Can you work these out from the model? Positions are in its coordinate system, mm. A direction names the side the tool comes from. Round coordinates to 2 decimals unless told otherwise and drop trailing zeros. Order: outer loops, then holes, each group sorted by start corner. A loop starts at its lowest first (then second) coordinate and runs counter-clockwise, first axis right, second up. Notation, with made-up numbers: (85.5, -9) -> (96.5, -9) arc R7 ccw to (96.5, 3) -> close; hole circle Ø11 at (-19, 31.25). An arc over 180 degrees is marked (long way). Use a Markdown table: item, result. Add a question column.
Q1. If we section it at D-D on y = 1.5: Give the number of separate pieces and of enclosed holes in the cut face, plus the area to 3 significant figures.
Q2. I'm going to push flat-ended pins straight in: pin 1 Ø3 at (y, z) = (7.5, 9) entering from +X; pin 2 Ø6 at (x, z) = (17.15, 0) entering from +Y; pin 3 Ø4 at (x, z) = (29.5, 20) entering from +Y. Where does each tip first touch, or does it pass through?
Q3. For faces 1 (the face through (7.324, 1.42, 23.396)), 2 (the face through (21, 14, -3)), 3 (the face through (30, 2.8, -23)), 4 (the face through (15.53, 10.8, -0.51)), 5 (the face through (62, 23, 23.25)), which set-ups out of +Z, -Z, +X, -X, +Y, -Y let a thin tool reach every point of the face, with its end or its side?
Q4. We'd pull the mould along Y, two halves only. Please class faces 6 (the face through (62, 14, -26.25)), 7 (the face through (119.196, 1.42, -21.738)), 8 (the face through (47.7, 0, -13)), 9 (the face through (62, 25.3, 27)): +Y half, -Y half, draft (parallel to the pull), parting line (faces both ways), or undercut.
Q5. I need wall thicknesses on line 1 along Z through (x, y) = (116, 20); line 2 along X through (y, z) = (1.1, -21.25); line 3 along X through (y, z) = (5.6, 21.25). Which ranges of each line are inside material? Lowest first, please. Write a range as [from, to].
Q6. If we section it at B-B on x = 62.5: List the corners of the cut face in (y, z) for me, plus the area to 3 significant figures.
Q7. If we section it at C-C on z = 0: List the corners of the cut face in (x, y) for me.
Q8. If we section it at A-A on y = 15: List the corners of the cut face in (x, z) for me.
```python
from build123d import *

# Parameters (mm, degrees)
BOSS_EXTRUDE1_DEPTH                                 = 125
CUT_EXTRUDE1_REACH                                  = 133.073
SKETCH4_R                                           = 19.5
SKETCH4_R_2                                         = 2.9
CUT_EXTRUDE2_DEPTH                                  = 132.07308076
CUT_EXTRUDE2_DEPTH_BACK                             = 132.07308076
SKETCH4_2_R                                         = 2.9
CBORE_FOR_M4_HEX_SOCKET_HEAD_CAP_SCR_2_COUNT        = 2
CBORE_FOR_M4_HEX_SOCKET_HEAD_CAP_SCR_2_PITCH        = 42.5
CBORE_FOR_M4_HEX_SOCKET_HEAD_CAP_SCR_3_COUNT        = 2
CBORE_FOR_M4_HEX_SOCKET_HEAD_CAP_SCR_3_PITCH        = 116.992521128
CBORE_FOR_M4_HEX_SOCKET_HEAD_CAP_SCR_4_COUNT        = 2
CBORE_FOR_M4_HEX_SOCKET_HEAD_CAP_SCR_4_PITCH        = 109
CBORE_FOR_M4_HEX_SOCKET_HEAD_CAP_SCR_5_COUNT        = 2
CBORE_FOR_M4_HEX_SOCKET_HEAD_CAP_SCR_5_PITCH        = 89
CBORE_FOR_M4_HEX_SOCKET_HEAD_CAP_SCR_6_COUNT        = 2
CBORE_FOR_M4_HEX_SOCKET_HEAD_CAP_SCR_6_PITCH        = 20
CBORE_FOR_M4_HEX_SOCKET_HEAD_CAP_SCR_7_COUNT        = 2
CBORE_FOR_M4_HEX_SOCKET_HEAD_CAP_SCR_7_PITCH        = 46.97073557
CBORE_FOR_M4_HEX_SOCKET_HEAD_CAP_SCR_8_COUNT        = 2
CBORE_FOR_M4_HEX_SOCKET_HEAD_CAP_SCR_8_PITCH        = 98.62682191
CBORE_FOR_M3_HEX_SOCKET_HEAD_CAP_SCREW1_D           = 3.4
CBORE_FOR_M3_HEX_SOCKET_HEAD_CAP_SCREW1_CBORE_D     = 6.5
CBORE_FOR_M3_HEX_SOCKET_HEAD_CAP_SCREW1_CBORE_DEPTH = 3.4


with BuildPart() as part:
    # Sketch2 → Boss-Extrude1 (new body)
    with BuildSketch(Plane(origin=(0, 0, 0), x_dir=(0, 0, -1), z_dir=(1, 0, 0))):
        Polygon((0, 0), (-30.25, 0), (-30.25, 25.3), (-23.25, 25.3), (-23.25, 21.3), (-26.25, 21.3), (-26.25, 7), (-3, 7), (-3, 21.3), (-9, 21.3), (-9, 25.3), (0, 25.3), align=None)
    boss_extrude1 = extrude(amount=BOSS_EXTRUDE1_DEPTH)

    # Mirror1: Boss-Extrude1 across plane
    add(boss_extrude1.mirror(Plane.XY))

    # Cut-Extrude1: up to this face of the body (flat: up to its plane)
    cut_extrude1_end = Plane(part.part.faces().sort_by_distance((62.5, 21.3, 6))[0])
    # Sketch4 → Cut-Extrude1 (cut, up to the picked face)
    with BuildSketch(Plane(origin=(0, 0, 0), x_dir=(-1, 0, 0), z_dir=(0, -1, 0)), mode=Mode.PRIVATE) as cut_extrude1_sk1:
        with Locations(Location((-62.5, 0, 0), (0, 0, 90))):
            Circle(SKETCH4_R)
        with Locations(Location((-62.5, 0, 0), (0, 0, 90))):
            Circle(SKETCH4_R_2, mode=Mode.SUBTRACT)
    cut_extrude1_tool1 = split(extrude(cut_extrude1_sk1.sketch, amount=-CUT_EXTRUDE1_REACH, mode=Mode.PRIVATE), bisect_by=cut_extrude1_end, keep=Keep.BOTH, mode=Mode.PRIVATE)
    add(cut_extrude1_tool1.solids().sort_by(Axis((62.5, 0, 18.948457), (0, 1, 0)))[0], mode=Mode.SUBTRACT)

    # Sketch4<2> → Cut-Extrude2 (cut, two sides: drawn at the far end of the back side and taken through both)
    with BuildSketch(Plane(origin=(0, 0, 0), x_dir=(-1, 0, 0), z_dir=(0, -1, 0)).offset(-CUT_EXTRUDE2_DEPTH_BACK)):
        with Locations(Location((-62.5, 0, 0), (0, 0, 90))):
            Circle(SKETCH4_2_R)
    extrude(amount=CUT_EXTRUDE2_DEPTH + CUT_EXTRUDE2_DEPTH_BACK, mode=Mode.SUBTRACT)

    # Sketch6 → CBORE for M4 Hex Socket Head Cap Screw1 (revolve, cut)
    with BuildSketch(Plane(origin=(117, 7, 21.25), x_dir=(0, 0, 1), z_dir=(1, 0, 0))):
        Polygon((0, 0), (0, 7), (2.25, 7), (2.25, 4.2), (4, 4.2), (4, 0.025), (4.025, 0), align=None)
    cbore_for_m4_hex_socket_head_cap_screw1 = revolve(axis=Axis((117, 13.35, 21.25), (0, -1, 0)), mode=Mode.SUBTRACT)

    # CBORE for M4 Hex Socket Head Cap Scr 2: CBORE for M4 Hex Socket Head Cap Screw1 ×2
    with Locations(*[(0, 0, -i * CBORE_FOR_M4_HEX_SOCKET_HEAD_CAP_SCR_2_PITCH) for i in range(1, CBORE_FOR_M4_HEX_SOCKET_HEAD_CAP_SCR_2_COUNT)]):
        add(cbore_for_m4_hex_socket_head_cap_screw1, mode=Mode.SUBTRACT)

    # CBORE for M4 Hex Socket Head Cap Scr 3: CBORE for M4 Hex Socket Head Cap Screw1 ×2
    with Locations(*[Vector(-0.9316834866759449, 0, -0.3632710842543822) * (i * CBORE_FOR_M4_HEX_SOCKET_HEAD_CAP_SCR_3_PITCH) for i in range(1, CBORE_FOR_M4_HEX_SOCKET_HEAD_CAP_SCR_3_COUNT)]):
        add(cbore_for_m4_hex_socket_head_cap_screw1, mode=Mode.SUBTRACT)

    # CBORE for M4 Hex Socket Head Cap Scr 4: CBORE for M4 Hex Socket Head Cap Screw1 ×2
    with Locations(*[(-i * CBORE_FOR_M4_HEX_SOCKET_HEAD_CAP_SCR_4_PITCH, 0, 0) for i in range(1, CBORE_FOR_M4_HEX_SOCKET_HEAD_CAP_SCR_4_COUNT)]):
        add(cbore_for_m4_hex_socket_head_cap_screw1, mode=Mode.SUBTRACT)

    # CBORE for M4 Hex Socket Head Cap Scr 5: CBORE for M4 Hex Socket Head Cap Screw1 ×2
    with Locations(*[(-i * CBORE_FOR_M4_HEX_SOCKET_HEAD_CAP_SCR_5_PITCH, 0, 0) for i in range(1, CBORE_FOR_M4_HEX_SOCKET_HEAD_CAP_SCR_5_COUNT)]):
        add(cbore_for_m4_hex_socket_head_cap_screw1, mode=Mode.SUBTRACT)

    # CBORE for M4 Hex Socket Head Cap Scr 6: CBORE for M4 Hex Socket Head Cap Screw1 ×2
    with Locations(*[(-i * CBORE_FOR_M4_HEX_SOCKET_HEAD_CAP_SCR_6_PITCH, 0, 0) for i in range(1, CBORE_FOR_M4_HEX_SOCKET_HEAD_CAP_SCR_6_COUNT)]):
        add(cbore_for_m4_hex_socket_head_cap_screw1, mode=Mode.SUBTRACT)

    # CBORE for M4 Hex Socket Head Cap Scr 7: CBORE for M4 Hex Socket Head Cap Screw1 ×2
    with Locations(*[Vector(-0.4257970363298798, 0, -0.904818702200994) * (i * CBORE_FOR_M4_HEX_SOCKET_HEAD_CAP_SCR_7_PITCH) for i in range(1, CBORE_FOR_M4_HEX_SOCKET_HEAD_CAP_SCR_7_COUNT)]):
        add(cbore_for_m4_hex_socket_head_cap_screw1, mode=Mode.SUBTRACT)

    # CBORE for M4 Hex Socket Head Cap Scr 8: CBORE for M4 Hex Socket Head Cap Screw1 ×2
    with Locations(*[Vector(-0.9023914415646597, 0, -0.43091726142132625) * (i * CBORE_FOR_M4_HEX_SOCKET_HEAD_CAP_SCR_8_PITCH) for i in range(1, CBORE_FOR_M4_HEX_SOCKET_HEAD_CAP_SCR_8_COUNT)]):
        add(cbore_for_m4_hex_socket_head_cap_screw1, mode=Mode.SUBTRACT)

    # CBORE for M3 Hex Socket Head Cap Screw1 (through all)
    with Locations(Plane(origin=(0, 25.3, 0), x_dir=(1, 0, 0), z_dir=(0, 1, 0))):
        with Locations((87.849101299, 0), (17.150898701, 0)):
            CounterBoreHole(CBORE_FOR_M3_HEX_SOCKET_HEAD_CAP_SCREW1_D / 2, CBORE_FOR_M3_HEX_SOCKET_HEAD_CAP_SCREW1_CBORE_D / 2, CBORE_FOR_M3_HEX_SOCKET_HEAD_CAP_SCREW1_CBORE_DEPTH)


solid = part.part
```
Answer below:
| question | item | result |
|---|---|---|
| 1 | separate pieces | 1 |
| 1 | enclosed holes | 11 |
| 1 | area | 6,220 mm² |
| 2 | pin 1 | x = 125 |
| 2 | pin 2 | y = 21.9 |
| 2 | pin 3 | y = 2.8 |
| 3 | face 1 | -Y |
| 3 | face 2 | +X, -X |
| 3 | face 3 | none |
| 3 | face 4 | +Y, -Y |
| 3 | face 5 | +X, -X, +Y |
| 4 | face 6 | undercut |
| 4 | face 7 | draft |
| 4 | face 8 | -Y half |
| 4 | face 9 | +Y half |
| 5 | line 1 | [-30.25, -26.25], [-3, 3], [26.25, 30.25] |
| 5 | line 2 | [0, 5.75], [10.25, 25.75], [30.25, 94.75], [99.25, 114.75], [119.25, 125] |
| 5 | line 3 | [0, 4], [12, 24], [32, 93], [101, 113], [121, 125] |
| 6 | outline | (0, -30.25) -> (25.3, -30.25) -> (25.3, -23.25) -> (21.3, -23.25) -> (21.3, -26.25) -> (7, -26.25) -> (7, -19.5) -> (0, -19.5) -> close; (0, 19.5) -> (7, 19.5) -> (7, 26.25) -> (21.3, 26.25) -> (21.3, 23.25) -> (25.3, 23.25) -> (25.3, 30.25) -> (0, 30.25) -> close; (21.3, -9) -> (25.3, -9) -> (25.3, -2.9) -> (21.3, -2.9) -> close; (21.3, 2.9) -> (25.3, 2.9) -> (25.3, 9) -> (21.3, 9) -> close |
| 6 | area | 370 mm² |
| 7 | outline | (0, 0) -> (15.45, 0) -> (15.45, 21.9) -> (13.9, 21.9) -> (13.9, 25.3) -> (0, 25.3) -> close; (18.85, 0) -> (43, 0) -> (43, 21.3) -> (59.6, 21.3) -> (59.6, 25.3) -> (20.4, 25.3) -> (20.4, 21.9) -> (18.85, 21.9) -> close; (65.4, 21.3) -> (82, 21.3) -> (82, 0) -> (86.15, 0) -> (86.15, 21.9) -> (84.6, 21.9) -> (84.6, 25.3) -> (65.4, 25.3) -> close; (89.55, 0) -> (125, 0) -> (125, 25.3) -> (91.1, 25.3) -> (91.1, 21.9) -> (89.55, 21.9) -> close |
| 8 | outline | (0, -30.25) -> (125, -30.25) -> (125, -26.25) -> (0, -26.25) -> close; (0, -3) -> (43.23, -3) arc R19.5 cw to (43.23, 3) -> (0, 3) -> close; (0, 26.25) -> (125, 26.25) -> (125, 30.25) -> (0, 30.25) -> close; (81.77, -3) -> (125, -3) -> (125, 3) -> (81.77, 3) arc R19.5 cw to start; hole circle Ø3.4 at (17.15, 0); hole circle Ø3.4 at (87.85, 0) |
